```python
from build123d import *

# Parameters (mm, degrees)
SKETCH_1_W        = 40
SKETCH_1_H        = 80
EXTRUDE_1_DEPTH   = 2
CHAMFER_1_SIZE    = 2
HOLE_WIZARD_M81_D = 9


with BuildPart() as part:
    # Эскиз1 → Бобышка-Вытянуть1 (new body)
    with BuildSketch(Plane.XY):
        Rectangle(SKETCH_1_W, SKETCH_1_H)
    extrude(amount=EXTRUDE_1_DEPTH)

    # Фаска1
    chamfer_1_edges = [part.edges().sort_by_distance(p)[0] for p in [
        (20, -40, 1),
        (-20, -40, 1),
        (-20, 40, 1),
        (20, 40, 1),
    ]]
    chamfer(chamfer_1_edges, length=CHAMFER_1_SIZE)

    # Отверстие с зазором M81 (through all)
    with Locations(Plane.XY.offset(2)):
        with Locations((0, -20), (0, 20)):
            Hole(HOLE_WIZARD_M81_D / 2)


solid = part.part
```
Model file for the job. Use its own axes, mm. Give positions to 0.01 mm unless a question says otherwise; leave off trailing zeros. Loops run counter-clockwise (first coordinate to the right, second up) from the corner with the lowest first, then second, coordinate; pieces in that order, holes last. Notation, with made-up numbers: (13, -7.75) - (64, -7.75) arc R16 ccw to (64, -1.75) - close; hole circle Ø4 at (-32, -33). An arc over 180 degrees is marked (long way). One line per item, written item: value. Start each with the question number.
1. Slice it at C-C (z = 0.9). List the corners of the cut face in (x, y).
2. Pull direction Y, two halves, no side cores. Call faces 1 (the cylindrical face through (0.59, -15.54, 0.99)), 2 (the flat face through (-19, -39, 1)), 3 (the flat face through (-20, -1, 1)), 4 (the cylindrical face through (-2.419, 23.794, 0.986)): pulls with the +Y half, pulls with the -Y half, needs draft (parallel to the pull), parting line crosses it, or undercut.
3. Probe L1, parallel to Y at x = 0, z = 1.4; L2, parallel to Y at x = 2, z = 1.6; L3, parallel to X at y = -21.5, z = 0.35. List the from-to ranges inside material, lowest first. Write a range as from..to.
4. Pin check, flat tip, straight feed: pin 1 (5.5 mm diameter, centred on x = 0, y = -20, fed in from +Z). Stop position of the tip, or through.
5. Slice it at B-B (y = -20). List the corners of the cut face in (x, z), plus the area to 3 significant figures.
6. Slice it at A-A (x = 0). List the corners of the cut face in (y, z).
Solution:
1. outline: (-20, -38) - (-18, -40) - (18, -40) - (20, -38) - (20, 38) - (18, 40) - (-18, 40) - (-20, 38) - close; hole circle Ø9 at (0, -20); hole circle Ø9 at (0, 20)
2. face 1: undercut
2. face 2: pulls with the -Y half
2. face 3: needs draft
2. face 4: undercut
3. L1: y = -40..-24.5, -15.5..15.5, 24.5..40
3. L2: y = -40..-24.03, -15.97..15.97, 24.03..40
3. L3: x = -20..-4.24, 4.24..20
4. pin 1: passes through
5. outline: (-20, 0) - (-4.5, 0) - (-4.5, 2) - (-20, 2) - close; (4.5, 0) - (20, 0) - (20, 2) - (4.5, 2) - close
5. area: 62.0 mm^2
6. outline: (-40, 0) - (-24.5, 0) - (-24.5, 2) - (-40, 2) - close; (-15.5, 0) - (15.5, 0) - (15.5, 2) - (-15.5, 2) - close; (24.5, 0) - (40, 0) - (40, 2) - (24.5, 2) - close
